Input: part model. Units: mm. Frame: model coordinates. Round coordinates to 2 decimals unless told otherwise and drop trailing zeros. Order: outer loops, then holes, each group sorted by start corner. A loop starts at its lowest first (then second) coordinate and runs counter-clockwise, first axis right, second up. Notation, with made-up numbers: (12.25, 71) - (23.25, 71) arc R10 cw to (23.25, 80) - close; hole circle Ø8 at (42, 67). An arc over 180 degrees is marked (long way). One line per item, written item: value. Start each with the question number.
from build123d import *

# Parameters (mm, degrees)
SKETCH1_R           = 5.3213
SKETCH1_R_2         = 2.1463
SKETCH1_R_3         = 12.827
SKETCH1_R_4         = 6.477
BOSS_EXTRUDE1_DEPTH = 2.54


with BuildPart() as part:
    # Sketch1 → Boss-Extrude1 (new body)
    # profile 1 of 5: a face of its own
    with BuildSketch(Plane(origin=(0, 0, 0), x_dir=(1, 0, 0), z_dir=(0, 1, 0))):
        with BuildLine():
            Line((-3.7903785, 12.25418132), (-26.97244415, 5.08366532))
            ThreePointArc((-26.97244415, 5.08366532), (-22.241773707, 4.282737486), (-20.0787, 0))
            ThreePointArc((-20.0787, 0), (-22.241773707, -4.282737486), (-26.97244415, -5.08366532))
            Line((-26.97244415, -5.08366532), (-3.7903785, -12.25418132))
            ThreePointArc((-3.7903785, -12.25418132), (-12.827, 0), (-3.7903785, 12.25418132))
        make_face()
    # profile 2 of 5: a face of its own
    with BuildSketch(Plane(origin=(0, 0, 0), x_dir=(1, 0, 0), z_dir=(0, 1, 0))):
        with Locations((-25.4, 0)):
            Circle(SKETCH1_R)
        with Locations(Location((-25.4, 0, 0), (0, 0, 270))):
            Circle(SKETCH1_R_2, mode=Mode.SUBTRACT)
    # profile 3 of 5: a face of its own
    with BuildSketch(Plane(origin=(0, 0, 0), x_dir=(1, 0, 0), z_dir=(0, 1, 0))):
        Circle(SKETCH1_R_3)
        with Locations(Location((0, 0, 0), (0, 0, 270))):
            Circle(SKETCH1_R_4, mode=Mode.SUBTRACT)
    # profile 4 of 5: a face of its own
    with BuildSketch(Plane(origin=(0, 0, 0), x_dir=(1, 0, 0), z_dir=(0, 1, 0))):
        with BuildLine():
            Line((26.97244415, 5.08366532), (3.7903785, 12.25418132))
            ThreePointArc((3.7903785, 12.25418132), (10.32354382, 7.612908248), (12.827, 0))
            ThreePointArc((12.827, 0), (10.32354382, -7.612908248), (3.7903785, -12.25418132))
            Line((3.7903785, -12.25418132), (26.97244415, -5.08366532))
            ThreePointArc((26.97244415, -5.08366532), (20.0787, 0), (26.97244415, 5.08366532))
        make_face()
    # profile 5 of 5: a face of its own
    with BuildSketch(Plane(origin=(0, 0, 0), x_dir=(1, 0, 0), z_dir=(0, 1, 0))):
        with Locations((25.4, 0)):
            Circle(SKETCH1_R)
        with Locations(Location((25.4, 0, 0), (0, 0, 270))):
            Circle(SKETCH1_R_2, mode=Mode.SUBTRACT)
    extrude(amount=BOSS_EXTRUDE1_DEPTH)


solid = part.part
Item 1: Section query D-D on z = -3. Return loops of the section in (x, y), and give its area (3 significant figures).
Item 2: Section query C-C on y = 0.5. Return loops of the section in (x, z), and give its area (3 significant figures).
Item 3: Pull-direction query (X, two-part tool) for faces 1 (the face through (-15.22, 1.25, -8.72)), 2 (the face through (-7, 0, 0)), 3 (the face through (-27.495, 1.252, -0.465)); classes: released by +X, released by -X, zero draft, split by the parting line, or undercut.
Item 4: Section query A-A on x = 0. Return loops of the section in (y, z).
Item 5: Line query: L1, parallel to X at y = 0.85, z = 0; L2, parallel to Z at x = 1, y = 2.35; L3, parallel to Z at x = -3, y = 1.3. Output: solid intervals per line, ascending.
Item 6: Section query B-B on z = 0. Return loops of the section in (x, y).
Geometry results:
1. outline: (-29.8, 0) - (-5.74, 0) - (-5.74, 2.54) - (-29.8, 2.54) - close; (5.74, 0) - (29.8, 0) - (29.8, 2.54) - (5.74, 2.54) - close
1. area: 122 mm^2
2. outline: (-26.97, -5.08) - (-3.79, -12.25) arc R12.83 ccw to (3.79, -12.25) - (26.97, -5.08) arc R5.32 ccw to (26.97, 5.08) - (3.79, 12.25) arc R12.83 ccw to (-3.79, 12.25) - (-26.97, 5.08) arc R5.32 ccw to start; hole circle Ø4.29 at (-25.4, 0); hole circle Ø12.95 at (0, 0); hole circle Ø4.29 at (25.4, 0)
2. area: 891 mm^2
3. face 1: released by -X
3. face 2: zero draft
3. face 3: undercut
4. outline: (0, -12.83) - (2.54, -12.83) - (2.54, -6.48) - (0, -6.48) - close; (0, 6.48) - (2.54, 6.48) - (2.54, 12.83) - (0, 12.83) - close
5. L1: x = -30.72 to -27.55, -23.25 to -6.48, 6.48 to 23.25, 27.55 to 30.72
5. L2: z = -12.79 to -6.4, 6.4 to 12.79
5. L3: z = -12.47 to -5.74, 5.74 to 12.47
6. outline: (-30.72, 0) - (-27.55, 0) - (-27.55, 2.54) - (-30.72, 2.54) - close; (-23.25, 0) - (-6.48, 0) - (-6.48, 2.54) - (-23.25, 2.54) - close; (6.48, 0) - (23.25, 0) - (23.25, 2.54) - (6.48, 2.54) - close; (27.55, 0) - (30.72, 0) - (30.72, 2.54) - (27.55, 2.54) - close
